Input: dimensioned drawing with shaded views. Units: mm. Origin: part minimum x, y, z. A direction names the side the tool comes from. Give positions to 0.01 mm unless a question says otherwise; leave off trailing zeros. Loops run counter-clockwise (first coordinate to the right, second up) from the corner with the lowest first, then second, coordinate; pieces in that order, holes last.
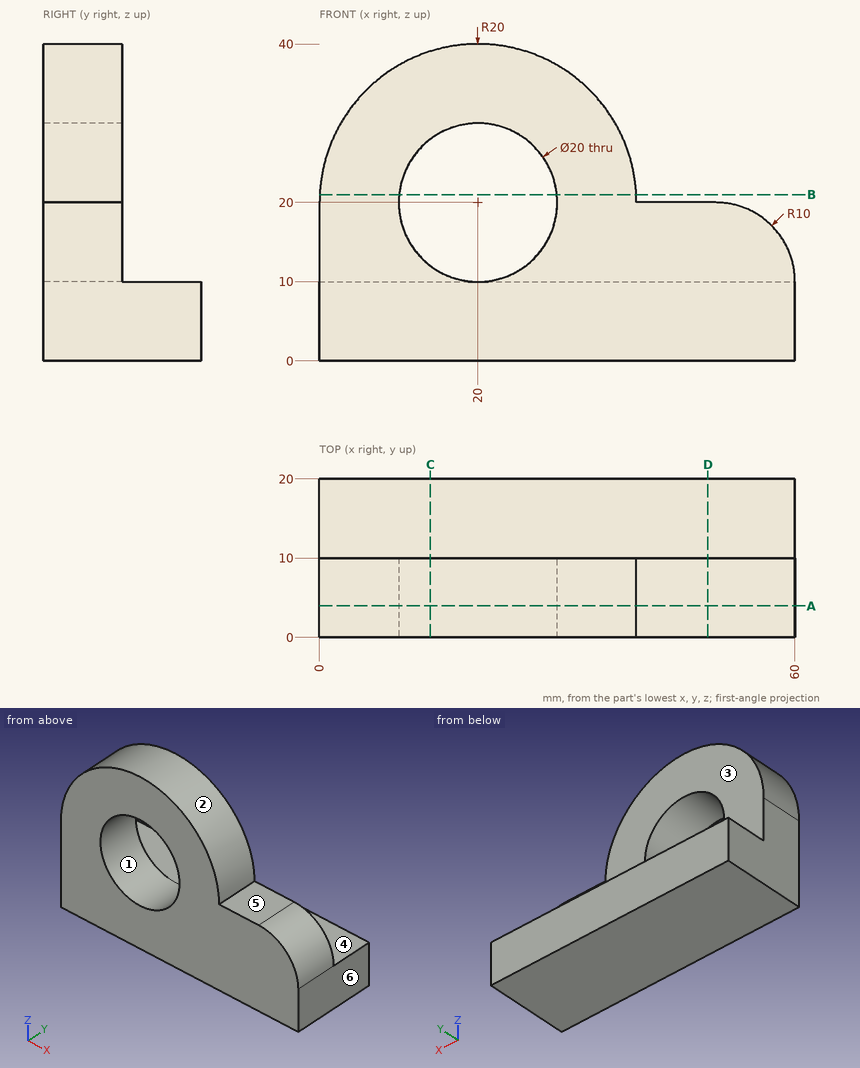
(1) Mould query, pull axis Z, two halves, no side actions, for the marked faces 1, 2 and 3. Classes: pulls with the +Z half, pulls with the -Z half, needs draft (parallel to the pull), parting line crosses it, or undercut.
A:
face 1: undercut
face 2: pulls with the +Z half
face 3: needs draft
(2) First-contact query: pin 1 (9 mm diameter, centred on x = 34.5, z = 18, fed in from +Y); pin 2 (12 mm diameter, centred on x = 49, y = 15, fed in from +Z); pin 3 (3 mm diameter, centred on x = 30.5, y = 14, fed in from +Z). Flat tips, straight axial feed; report the tip coordinate or a pass-through.
A:
pin 1: stops at y = 10
pin 2: stops at z = 20
pin 3: stops at z = 10
(3) Section A-A, the plane y = 4. Return the cut outline in (x, z).
A:
outline: (0, 0) - (60, 0) - (60, 10) arc R10 ccw to (50, 20) - (40, 20) arc R20 ccw to (0, 20) - close; hole circle Ø20 at (20, 20)
(4) Section D-D, the plane x = 49. Return the cut outline in (y, z), then the cut area to 3 significant figures.
A:
outline: (0, 0) - (20, 0) - (20, 10) - (10, 10) - (10, 20) - (0, 20) - close
area: 300 mm2
(5) Reachability of the marked faces 4, 5 and 6 from +Z, -Z, +X, -X, +Y, -Y: full face, straight path, thin tool, end or side. Return the list, or none.
A:
face 4: +Z, +X, -X, +Y
face 5: +Z, +X, +Y, -Y
face 6: +Z, -Z, +X, +Y, -Y
(6) Section B-B, the plane z = 21. Return the cut outline in (x, y), then the cut area to 3 significant figures.
A:
outline: (0.03, 0) - (10.05, 0) - (10.05, 10) - (0.03, 10) - close; (29.95, 0) - (39.97, 0) - (39.97, 10) - (29.95, 10) - close
area: 201 mm2
(7) Section C-C, the plane x = 14. Return the cut outline in (y, z), then the cut area to 3 significant figures.
A:
outline: (0, 0) - (20, 0) - (20, 10) - (10, 10) - (10, 12) - (0, 12) - close; (0, 28) - (10, 28) - (10, 39.08) - (0, 39.08) - close
area: 331 mm2
(8) Ray query, line 1 along Z through (x, y) = (20, 7); line 2 along Y through (x, z) = (35, 32); line 3 along X through (y, z) = (1, 24). Return the intervals inside material, ascending.
A:
line 1: z = 0 to 10, 30 to 40
line 2: y = 0 to 10
line 3: x = 0.4 to 10.83, 29.17 to 39.6
